Work out the finished part from the listing and answer in its coordinate system (mm). Coordinates: 2 decimals unless noted, no trailing zeros. Order: outer loops, then holes, each group sorted by start corner. A loop starts at its lowest first (then second) coordinate and runs counter-clockwise, first axis right, second up.
1. The part is cut by section C-C, the plane x = -46. Give the vertices of the cut face in (y, z).
2. The part is cut by section B-B, the plane z = 0. Give the vertices of the cut face in (x, y), then the cut area to 3 significant figures.
3. Flat-ended cylindrical pins translate along their axes: pin 1 Ø3 at (y, z) = (4, -20.5) entering from +X; pin 2 Ø4.5 at (x, z) = (0, -101.6) entering from -Y; pin 3 Ø2 at (x, z) = (-87.99, 50.8) entering from +Y; pin 4 Ø1 at (y, z) = (4, 17) entering from -X. Find the tip coordinate at first contact, or state that the pin passes through.
4. Determine the mould class of faces 1 (the cylindrical face through (-21.4, 2.5, 96.2)), 2 (the cylindrical face through (-88.286, 2.504, 67.695)), 3 (the flat face through (-8.8, 0, 98.4)) for opening direction X: +X half, -X half, draft (parallel to the pull), parting line (faces both ways), or undercut.
5. The part is cut by section A-A, the plane y = 3.4. Give the vertices of the cut face in (x, z).
6. Find the intervals of material crossed by probe 1 along Z at (x, y) = (0, 1.45); probe 2 along X at (y, z) = (2.1, -50.8); probe 3 along Z at (x, y) = (3, 4.7), in increasing order.
```python
from build123d import *

# Parameters (mm, degrees)
SKETCH1_R                     = 111.252
SKETCH1_R_2                   = 98.552
BOSS_EXTRUDE1_DEPTH           = 5.08
TAP_DRILL_FOR_8_32_TAP1_D     = 3.4544
TAP_DRILL_FOR_8_32_TAP1_DEPTH = 25.4
TAP_DRILL_FOR_8_32_TAP1_TIP   = 1.037806461


with BuildPart() as part:
    # Sketch1 → Boss-Extrude1 (new body)
    with BuildSketch(Plane(origin=(0, 0, 0), x_dir=(1, 0, 0), z_dir=(0, 1, 0))):
        Circle(SKETCH1_R)
        Circle(SKETCH1_R_2, mode=Mode.SUBTRACT)
    extrude(amount=BOSS_EXTRUDE1_DEPTH)

    # Tap Drill for #8-32 Tap1
    with Locations(Plane(origin=(0, 5.08, 0), x_dir=(1, 0, 0), z_dir=(0, 1, 0))):
        with Locations((-87.988181024, 50.8), (0, 101.6), (87.988181024, 50.8), (87.988181024, -50.8), (0, -101.6), (-87.988181024, -50.8)):
            Hole(TAP_DRILL_FOR_8_32_TAP1_D / 2, depth=TAP_DRILL_FOR_8_32_TAP1_DEPTH)
            with Locations((0, 0, -(TAP_DRILL_FOR_8_32_TAP1_DEPTH + TAP_DRILL_FOR_8_32_TAP1_TIP / 2))):  # 118° drill point
                Cone(0, TAP_DRILL_FOR_8_32_TAP1_D / 2, TAP_DRILL_FOR_8_32_TAP1_TIP, mode=Mode.SUBTRACT)


solid = part.part
```
Geometry says:
1. outline: (0, -101.3) - (5.08, -101.3) - (5.08, -87.16) - (0, -87.16) - close; (0, 87.16) - (5.08, 87.16) - (5.08, 101.3) - (0, 101.3) - close
2. outline: (-111.25, 0) - (-98.55, 0) - (-98.55, 5.08) - (-111.25, 5.08) - close; (98.55, 0) - (111.25, 0) - (111.25, 5.08) - (98.55, 5.08) - close
2. area: 129 mm2
3. pin 1: stops at x = 109.62
3. pin 2: stops at y = 0
3. pin 3: passes through
3. pin 4: stops at x = -110.02
4. face 1: undercut
4. face 2: parting line
4. face 3: draft
5. outline: circle Ø222.5 at (0, 0); hole circle Ø197.1 at (0, 0); hole circle Ø3.45 at (-87.99, -50.8); hole circle Ø3.45 at (-87.99, 50.8); hole circle Ø3.45 at (0, -101.6); hole circle Ø3.45 at (0, 101.6); hole circle Ø3.45 at (87.99, -50.8); hole circle Ø3.45 at (87.99, 50.8)
6. probe 1: z = -111.25 to -103.33, -99.87 to -98.55, 98.55 to 99.87, 103.33 to 111.25
6. probe 2: x = -98.98 to -89.72, -86.26 to -84.45, 84.45 to 86.26, 89.72 to 98.98
6. probe 3: z = -111.21 to -98.51, 98.51 to 111.21
